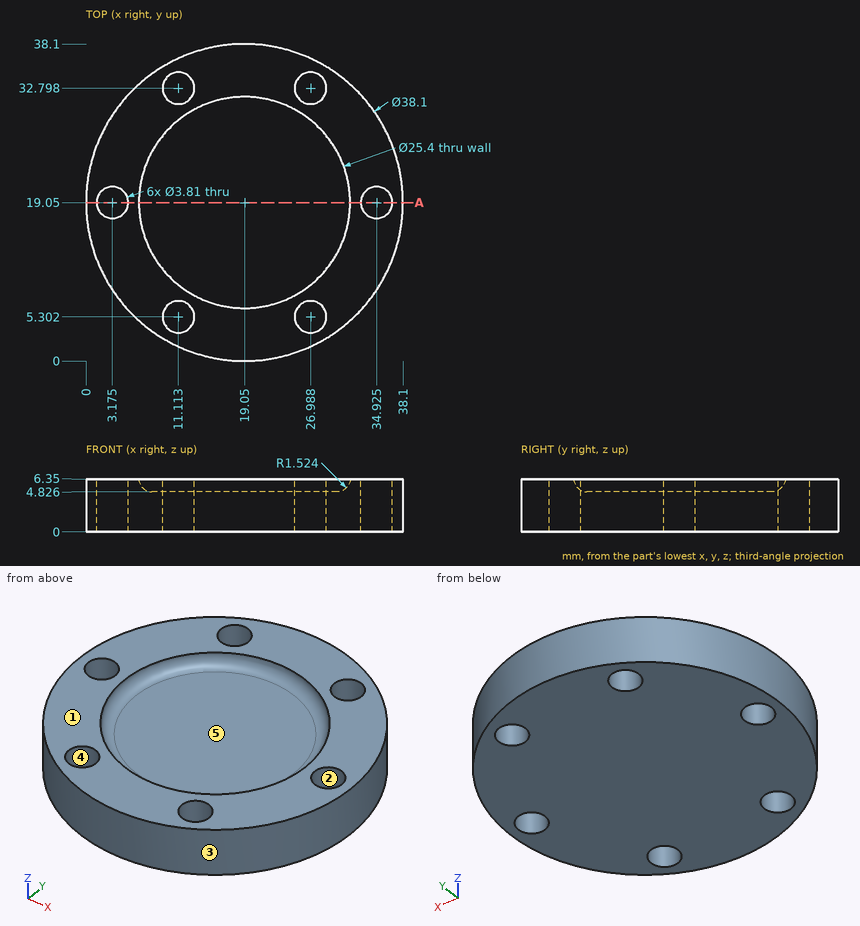
Part print with two shaded views. Sizes in mm from the minimum x, y, z corner. A direction names the side the tool comes from. Coordinates: 2 decimals unless noted, no trailing zeros. Put each result on its own line as item: value.
1. Two-plate mould, pull along Y, no slides. Class the marked faces 1, 2 and 3: +Y half, -Y half, draft (parallel to the pull), parting line (faces both ways), or undercut.
Final values:
face 1: draft
face 2: undercut
face 3: parting line
2. Band-saw the part on A-A (y = 19.05). Give the number of separate pieces and of enclosed holes in the cut face, then the cut area to 3 significant figures.
Final values:
separate pieces: 3
enclosed holes: 0
area: 156 mm²
3. Flat gauge pins, fed straight in: pin 1 Ø1.5 at (y, z) = (15, 4) entering from -X; pin 2 Ø2.5 at (x, y) = (11.11, 5.3) entering from -Z; pin 3 Ø2 at (x, z) = (13.5, 4.5) entering from +Y; pin 4 Ø1 at (x, y) = (30, 17.5) entering from +Z (1 decimal). Where does each tip first touch, or does it go through?
Final values:
pin 1: stops at x = 0.29
pin 2: passes through
pin 3: stops at y = 37.55
pin 4: stops at z = 4.9
4. 3-axis set-ups, long thin cutter, end or side, ignore diameter. For the marked faces 4 and 5: which of +Z, -Z, +X, -X, +Y, -Y reach the whole face in a straight line?
Final values:
face 4: +Z, -Z
face 5: +Z
5. Probe line 1 along Y through (x, z) = (26, 3.75) (1 decimal); line 2 along X through (y, z) = (31.5, 0.5) (1 decimal); line 3 along X through (y, z) = (18, 4.75) (1 decimal). List the from-to ranges inside material, lowest first. Write a range as [from, to].
Final values:
line 1: y = [1.3, 3.7], [6.9, 31.2], [34.4, 36.8]
line 2: x = [4.6, 9.7], [12.5, 25.6], [28.4, 33.5]
line 3: x = [0, 1.6], [4.8, 33.3], [36.5, 38.1]
